from build123d import *

# Parameters (mm, degrees)
SKETCH1_W               = 2.5
SKETCH1_H               = 2.25
SKETCH2_R               = 1.25
BOSS_EXTRUDE1_DEPTH     = 8
CUT_EXTRUDE1_DEPTH      = 1.1
CHAMFER1_SIZE           = 0.2535
FILLET1_R               = 0.125
SKETCH5_W               = 5
SKETCH5_H               = 4.609791228
CUT_EXTRUDE2_DEPTH      = 10
CUT_EXTRUDE2_DEPTH_BACK = 10


with BuildPart() as part:
    # Sketch1 → Revolve1 (revolve)
    with BuildSketch(Plane(origin=(0, 0, 0), x_dir=(-1, 0, 0), z_dir=(0, 0, -1))):
        with Locations((-1.25, 1.125)):
            Rectangle(SKETCH1_W, SKETCH1_H)
    revolve(axis=Axis((2.5, 0, 0), (-1, 0, 0)))

    # Sketch2 → Boss-Extrude1 (add)
    with BuildSketch(Plane(origin=(2.5, 0, 0), x_dir=(0, 0, -1), z_dir=(1, 0, 0))):
        Circle(SKETCH2_R)
    extrude(amount=BOSS_EXTRUDE1_DEPTH)

    # Sketch3 → Cut-Extrude1 (cut)
    with BuildSketch(Plane.ZY):
        Polygon((-1.0225, -0.59034065), (0, -1.1806813), (1.0225, -0.59034065), (1.0225, 0.59034065), (0, 1.1806813), (-1.0225, 0.59034065), align=None)
    extrude(amount=-CUT_EXTRUDE1_DEPTH, mode=Mode.SUBTRACT)

    # Sketch4 → Cut-Revolve1 (revolve, cut)
    with BuildSketch(Plane.XY):
        Polygon((1.1, 1.0225), (1.1, 0), (1.69034065, 0), align=None)
    revolve(axis=Axis((1.099975, 0, 0), (1, 0, 0)), mode=Mode.SUBTRACT)

    # Chamfer1
    chamfer1_edges = [part.edges().sort_by_distance(p)[0] for p in [
        (10.5, 0, 1.25),
    ]]
    chamfer(chamfer1_edges, length=CHAMFER1_SIZE)

    # Fillet1
    fillet1_edges = [part.edges().sort_by_distance(p)[0] for p in [
        (0, -2.25, 0),
        (2.5, 0, 1.25),
    ]]
    fillet(fillet1_edges, radius=FILLET1_R)

    # Sketch5 → Cut-Extrude2 (cut, two sides)
    with BuildSketch(Plane.XY) as cut_extrude2_sk:
        with Locations((8, -0.404062901)):
            Rectangle(SKETCH5_W, SKETCH5_H)
    extrude(amount=CUT_EXTRUDE2_DEPTH, mode=Mode.SUBTRACT)
    extrude(cut_extrude2_sk.sketch, amount=-CUT_EXTRUDE2_DEPTH_BACK, mode=Mode.SUBTRACT)


solid = part.part
Could you check a few things on this model? Use its own coordinates, in mm. A direction names the side the tool comes from. Give positions to 0.01 mm unless a question says otherwise; leave off trailing zeros. Order: outer loops, then holes, each group sorted by start corner. A loop starts at its lowest first (then second) coordinate and runs counter-clockwise, first axis right, second up.
1. I need wall thicknesses on L1, parallel to X at y = 1.7, z = 0.25; L2, parallel to Z at x = 1.05, y = 0; L3, parallel to Z at x = 0.55, y = 1.1. Which ranges of each line are inside material? Lowest first, please.
2. We'd pull the mould along Z, two halves only. Please class faces 4 (the cylindrical face through (4.04, -1.22, 0.27)), 5 (the flat face through (5.5, 0, 0)), 6 (the flat face through (0.54, 0.88, 0.52)): pulls with the +Z half, pulls with the -Z half, needs draft (parallel to the pull), parting line crosses it, or undercut.
3. For faces 1 (the flat face through (0.54, 0.89, -0.5)), 2 (the flat face through (2.5, -0.5, 1.5)), 3 (the cylindrical face through (1.3, -0.29, -2.23)), which set-ups out of +Z, -Z, +X, -X, +Y, -Y let a thin tool reach every point of the face, with its end or its side?
4. Suppose I cut it at C-C (x = 3.35). List the corners of the cut face in (y, z) for me.
5. Suppose I cut it at B-B (x = 2.1). List the corners of the cut face in (y, z) for me.
6. Suppose I cut it at A-A (x = 0.9). List the corners of the cut face in (y, z) for me.
7. Will these pins go through, and if not, where does the flat tip stop? P1, Ø1.5, axis at x = 2, z = 1, coming from the +Y side; P2, Ø2, axis at x = 5, y = 1.5, coming from the -Z side; P3, Ø1.5, axis at x = 1.5, z = 1.5, coming from the +Y side.
Solved:
1. L1: x = 0 to 2.5
1. L2: z = -2.25 to -1.02, 1.02 to 2.25
1. L3: z = -1.96 to -0.14, 0.14 to 1.96
2. face 4: parting line crosses it
2. face 5: needs draft
2. face 6: undercut
3. face 1: -X
3. face 2: +X
3. face 3: +X, -X
4. outline: circle Ø2.5 at (0, 0)
5. outline: circle Ø4.5 at (0, 0)
6. outline: circle Ø4.5 at (0, 0); hole (-1.18, 0) - (-0.59, -1.02) - (0.59, -1.02) - (1.18, 0) - (0.59, 1.02) - (-0.59, 1.02) - close
7. P1: stops at y = 2.24
7. P2: stops at z = -1.15
7. P3: stops at y = 2.12
